Read the model definition and answer for the solid it produces. Units are mm, in the model's axes. A direction names the side the tool comes from. Round coordinates to 2 decimals unless told otherwise and drop trailing zeros. Order: outer loops, then holes, each group sorted by start corner. A loop starts at its lowest first (then second) coordinate and runs counter-clockwise, first axis right, second up.
from build123d import *

# Parameters (mm, degrees)
SKETCH1_R               = 2.1
BOSS_EXTRUDE1_DEPTH     = 10
SHELL2_T                = -3
SKETCH2_R               = 2.1
BOSS_EXTRUDE2_DEPTH     = 7.4
SKETCH3_W               = 5.2
SKETCH3_H               = 14
CUT_EXTRUDE1_DEPTH      = 1
CUT_EXTRUDE1_DEPTH_BACK = 11


with BuildPart() as part:
    # Sketch1 → Boss-Extrude1 (new body)
    with BuildSketch(Plane.XY):
        with BuildLine():
            Line((-37.5, 8), (37.5, 8))
            ThreePointArc((37.5, 8), (45.5, 0), (37.5, -8))
            Line((37.5, -8), (-37.5, -8))
            ThreePointArc((-37.5, -8), (-45.5, 0), (-37.5, 8))
        make_face()
        with Locations((-37.5, 0)):
            Circle(SKETCH1_R, mode=Mode.SUBTRACT)
        with Locations((37.5, 0)):
            Circle(SKETCH1_R, mode=Mode.SUBTRACT)
    extrude(amount=BOSS_EXTRUDE1_DEPTH)

    # Shell2
    shell2_openings = [part.faces().sort_by_distance(p)[0] for p in [
        (0, 0, 0),
    ]]
    offset(amount=SHELL2_T, openings=shell2_openings, kind=Kind.INTERSECTION)

    # Sketch2 → Boss-Extrude2 (add, symmetric)
    with BuildSketch(Plane(origin=(0, 0, 0), x_dir=(0, 0, -1), z_dir=(1, 0, 0))):
        with BuildLine():
            Line((-10, -8), (-10, -16))
            ThreePointArc((-10, -16), (-6.46292884, -19.973121807), (-2.107151555, -16.919636334))
            Line((-2.107151555, -16.919636334), (0, -8))
            Line((0, -8), (-10, -8))
        make_face()
        with Locations((-6, -16)):
            Circle(SKETCH2_R, mode=Mode.SUBTRACT)
    extrude(amount=BOSS_EXTRUDE2_DEPTH, both=True)

    # Sketch3 → Cut-Extrude1 (cut, two sides)
    with BuildSketch(Plane.XY.offset(10)) as cut_extrude1_sk:
        with Locations((0, -15)):
            Rectangle(SKETCH3_W, SKETCH3_H)
    extrude(amount=CUT_EXTRUDE1_DEPTH, mode=Mode.SUBTRACT)
    extrude(cut_extrude1_sk.sketch, amount=-CUT_EXTRUDE1_DEPTH_BACK, mode=Mode.SUBTRACT)


solid = part.part
Q1. For a pull along X with two mould halves and no side action, classify faces 1 (the face through (7.4, -13, 5)), 2 (the face through (-2.6, -13, 5)), 3 (the face through (-1, 8, 5)) as released by +X, released by -X, zero draft, split by the parting line, or undercut.
Outcome:
face 1: released by +X
face 2: undercut
face 3: zero draft
Q2. Straight lines are drawn through the part: probe 1 along Y at (x, z) = (-4.2, 6); probe 2 along X at (y, z) = (-16.25, 3.75); probe 3 along Y at (x, z) = (37.5, 7). For each, find the intervals that lie inside material, in ascending order.
Outcome:
probe 1: y = -20 to -18.1, -13.9 to -5, 5 to 8
probe 2: x = -7.4 to -2.6, 2.6 to 7.4
probe 3: y = -8 to -2.1, 2.1 to 8
Q3. A cutting plane is placed at B-B, the plane y = 0. Give the vertices of the cut face in (x, z), plus the area to 3 significant figures.
Outcome:
outline: (-45.5, 0) - (-39.6, 0) - (-39.6, 10) - (-45.5, 10) - close; (-35.4, 0) - (-32.4, 0) - (-32.4, 7) - (32.4, 7) - (32.4, 0) - (35.4, 0) - (35.4, 10) - (-35.4, 10) - close; (39.6, 0) - (45.5, 0) - (45.5, 10) - (39.6, 10) - close
area: 372 mm2
Q4. A cutting plane is placed at C-C, the plane x = -4. Give the vertices of the cut face in (y, z).
Outcome:
outline: (-16.92, 2.11) - (-8, 0) - (-5, 0) - (-5, 7) - (5, 7) - (5, 0) - (8, 0) - (8, 10) - (-16, 10) arc R4 ccw to start; hole circle Ø4.2 at (-16, 6)
Q5. For faces 4 (the face through (-7.4, -13, 5)), 5 (the face through (23, -8, 5)), 6 (the face through (0, -8, 5)), 7 (the face through (-1, 5, 3)), determine the directions among +Z, -Z, +X, -X, +Y, -Y from which every point of the face is accessible in a straight line to the end or side of a thin tool.
Outcome:
face 4: +Z, -Z, -X, -Y
face 5: +Z, -Z, +X, -Y
face 6: +Z, -Z, -Y
face 7: -Z
Q6. Flat-ended cylindrical pins translate along their axes: pin 1 (1.6 mm diameter, centred on x = 1, z = 5.5, fed in from -Y); pin 2 (4 mm diameter, centred on y = -16, z = 6, fed in from +X); pin 3 (3 mm diameter, centred on y = -11.5, z = 3, fed in from -X); pin 4 (6 mm diameter, centred on y = 4, z = 1, fed in from -X). Find the tip coordinate at first contact, or state that the pin passes through.
Outcome:
pin 1: stops at y = -8
pin 2: passes through
pin 3: stops at x = -7.4
pin 4: stops at x = -45.44
Q7. A cutting plane is placed at A-A, the plane z = 6. Give the vertices of the cut face in (x, y), plus the area to 3 significant figures.
Outcome:
outline: (-37.5, -8) - (-7.4, -8) - (-7.4, -13.9) - (-2.6, -13.9) - (-2.6, -8) - (2.6, -8) - (2.6, -13.9) - (7.4, -13.9) - (7.4, -8) - (37.5, -8) arc R8 ccw to (37.5, 8) - (-37.5, 8) arc R8 ccw to start; (-7.4, -20) - (-2.6, -20) - (-2.6, -18.1) - (-7.4, -18.1) - close; (2.6, -20) - (7.4, -20) - (7.4, -18.1) - (2.6, -18.1) - close; hole circle Ø4.2 at (-37.5, 0); hole (-36.5, -5) - (36.5, -5) arc R5.1 cw to (36.5, 5) - (-36.5, 5) arc R5.1 cw to start; hole circle Ø4.2 at (37.5, 0)
area: 780 mm2
Q8. A cutting plane is placed at D-D, the plane x = 10. Give the vertices of the cut face in (y, z).
Outcome:
outline: (-8, 0) - (-5, 0) - (-5, 7) - (5, 7) - (5, 0) - (8, 0) - (8, 10) - (-8, 10) - close
